from build123d import *

# Parameters (mm, degrees)
SKETCH_1_R               = 3
EXTRUDE_1_DEPTH          = 4
CHAMFER_1_SIZE           = 0.5
SKETCH_4_R               = 4
EXTRUDE_2_DEPTH          = 8
HOLE_WIZARD_M4_2_D       = 3.3
HOLE_WIZARD_M4_2_DEPTH   = 10.1
HOLE_WIZARD_M4_2_TIP     = 0.991420021
CUT_EXTRUDE_1_DEPTH      = 10.797958971
CUT_EXTRUDE_1_DEPTH_BACK = 10.797958971
SKETCH_7_W               = 6.66597258
SKETCH_7_H               = 2.440047967


with BuildPart() as part:
    # 草图1 → 凸台-拉伸1 (new body)
    with BuildSketch(Plane.XY):
        Circle(SKETCH_1_R)
    extrude(amount=EXTRUDE_1_DEPTH)

    # 倒角1
    chamfer_1_edges = [part.edges().sort_by_distance(p)[0] for p in [
        (-3, 0, 4),
    ]]
    chamfer(chamfer_1_edges, length=CHAMFER_1_SIZE)

    # 草图4 → 凸台-拉伸2 (add)
    with BuildSketch(Plane(origin=(0, 0, 0), x_dir=(-1, 0, 0), z_dir=(0, 0, -1))):
        Circle(SKETCH_4_R)
    extrude(amount=EXTRUDE_2_DEPTH)

    # M4 螺纹孔2
    with Locations(Plane(origin=(0, 0, -8), x_dir=(-1, 0, 0), z_dir=(0, 0, -1))):
        with Locations((0, 0)):
            Hole(HOLE_WIZARD_M4_2_D / 2, depth=HOLE_WIZARD_M4_2_DEPTH)
            with Locations((0, 0, -(HOLE_WIZARD_M4_2_DEPTH + HOLE_WIZARD_M4_2_TIP / 2))):  # 118° drill point
                Cone(0, HOLE_WIZARD_M4_2_D / 2, HOLE_WIZARD_M4_2_TIP, mode=Mode.SUBTRACT)

    # 草图7 → 切除-拉伸1 (cut, two sides: drawn at the far end of the back side and taken through both)
    with BuildSketch(Plane(origin=(0, 0, 0), x_dir=(0, 0, -1), z_dir=(1, 0, 0)).offset(-CUT_EXTRUDE_1_DEPTH_BACK)):
        with Locations((2.66701371, 4.520023984)):
            Rectangle(SKETCH_7_W, SKETCH_7_H)
        with Locations((2.66701371, -4.520023984)):
            Rectangle(SKETCH_7_W, SKETCH_7_H)
    extrude(amount=CUT_EXTRUDE_1_DEPTH + CUT_EXTRUDE_1_DEPTH_BACK, mode=Mode.SUBTRACT)


solid = part.part
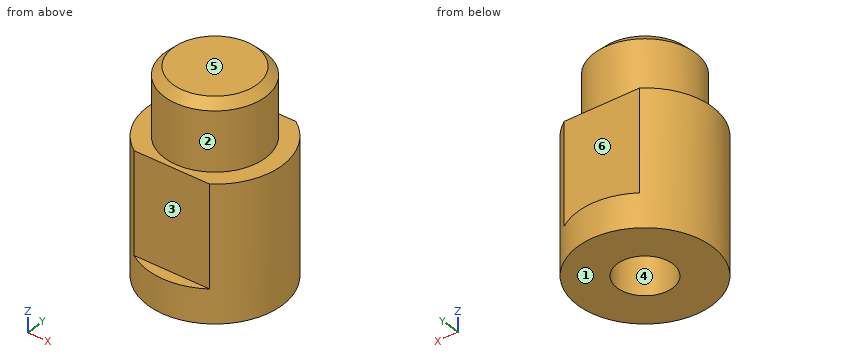
Geometry check sheet. Reference: the model listing, model coordinates, mm. Face numbers are marked on the shaded views. A direction names the side the tool comes from. Round coordinates to 2 decimals unless told otherwise and drop trailing zeros. Order: outer loops, then holes, each group sorted by start corner. A loop starts at its lowest first (then second) coordinate and runs counter-clockwise, first axis right, second up. Notation, with made-up numbers: M 4,4 L 24,4 A15 ccw 24,11 Z; hole C 12,10 d3. An arc over 180 degrees is marked long. Write each question's results on one line, items separated by ' | '. Start each with the question number.
1. Material ranges on L1, parallel to X at y = 0, z = -0.5; L2, parallel to Y at x = 0, z = -1; L3, parallel to Z at x = 1.75, y = -2.5, recorded low to high. Write a range as from..to.
2. Draft check along Y on the marked faces 4, 5 and 6. Enter one of: pulls with the +Y half, pulls with the -Y half, needs draft (parallel to the pull), parting line crosses it, or undercut.
3. Cross-section at D-D on z = 2.25. Record the boundary of the cut face in (x, y).
4. Cross-section at C-C on y = 3.75. Record the boundary of the cut face in (x, z), plus the area to 3 significant figures.
5. Cross-section at B-B on z = -7. Record the boundary of the cut face in (x, y), plus the area to 3 significant figures.
6. Set-up check for the marked faces 1, 2 and 3: record each of +Z, -Z, +X, -X, +Y, -Y from which the full face is reachable in a straight line by a thin tool's end or side.
7. Go/stop test with flat-tipped pins: P1, Ø0.6, axis at x = -0.5, y = 3.5, coming from the +Z side; P2, Ø4, axis at x = 2, z = -5, coming from the +Y side; P3, Ø3, axis at y = -2.5, z = 0.5, coming from the +X side. Record where each tip stops, or that it passes through.
8. Cross-section at A-A on z = -2.75. Record the boundary of the cut face in (x, y).
Resolved:
1) L1: -4..-1.65, 1.65..4 | L2: -3.3..-1.65, 1.65..3.3 | L3: -8..0
2) face 4: undercut | face 5: needs draft | face 6: pulls with the +Y half
3) outline: C 0,0 d6; hole C 0,0 d2.8
4) outline: M -1.39,-8 L 1.39,-8 L 1.39,-6 L -1.39,-6 Z | area: 5.57 mm2
5) outline: C 0,0 d8; hole C 0,0 d3.3 | area: 41.7 mm2
6) face 1: -Z, +X, -X, +Y, -Y | face 2: +Z | face 3: +Z, +X, -X, -Y
7) P1: z = 0 | P2: y = 3.99 | P3: x = 3.85
8) outline: M -2.26,-3.3 L 2.26,-3.3 A4 ccw 2.26,3.3 L -2.26,3.3 A4 ccw Z; hole C 0,0 d3.3
